For this review, take the finished solid that the model builds, in its own axes (mm). A direction names the side the tool comes from. Round coordinates to 2 decimals unless told otherwise and drop trailing zeros. Order: outer loops, then holes, each group sorted by start corner. A loop starts at its lowest first (then second) coordinate and runs counter-clockwise, first axis right, second up. Notation, with made-up numbers: (44, -32.75) -> (93, -32.75) arc R17 ccw to (93, -14.75) -> close; hole circle Ø7 at (60.25, 9). An arc over 180 degrees is marked (long way). Use a Markdown table: item, result. Add a question column.
1) Consider section D-D (x = 15.5). State the section outline as (y, z) points, plus the area to 3 significant figures.
2) Clearance check with flat-ended pins moving along their axes: P1, Ø10, axis at x = 23, y = -20, coming from the +Z side; P2, Ø5.5, axis at x = 19.5, z = 21, coming from the -Y side. State where each tip first meets the part, or that it passes through.
3) Consider section B-B (y = -3.5). State the section outline as (x, z) points.
4) Consider section C-C (x = 3). State the section outline as (y, z) points, plus the area to 3 significant figures.
5) Wall thickness on line 1 along X through (y, z) = (-9.5, 21); line 2 along Y through (x, z) = (29.5, 21); line 3 along Z through (x, y) = (30, -18.25): over which ranges is each line inside the solid? List them lowest first. Write a range as [from, to].
6) Draft analysis for pull direction X (two halves, no side actions). For faces 1 (the face through (19, -13, 0)), 2 (the face through (0, -10, 13)), 3 (the face through (12.7, -6, 25)), 4 (the face through (38.1, -10, 13)), state which applies: pulls with the +X half, pulls with the -X half, needs draft (parallel to the pull), parting line crosses it, or undercut.
7) Machinability: for faces 5 (the face through (19, -6, 19.05)), 6 (the face through (6, -6, 31.75)), 7 (the face through (19, -12.7, 18)), which of the approach directions +Z, -Z, +X, -X, +Y, -Y give a long, thin tool a straight path to every point of the face, cutting with its end or side? Answer none if there is none.
8) Consider section A-A (z = 30). State the section outline as (x, y) points.
```python
from build123d import *

# Parameters (mm, degrees)
F1_DEPTH = 38.1
F2_W     = 12.7
F2_H     = 12.7
F3_DEPTH = 228.6


with BuildPart() as f1:
    # F0 (on Right) → F1 (new body)
    with BuildSketch(Plane.YZ):
        Polygon((-25.4, 0), (0, 0), (0, 31.75), (-12.7, 31.75), (-12.7, 12.7), (-25.4, 12.7), align=None)
    extrude(amount=F1_DEPTH)

    # F2 (on Front) → F3 (cut)
    with BuildSketch(Plane.XZ):
        with Locations((19.05, 25.4)):
            Rectangle(F2_W, F2_H)
    extrude(amount=F3_DEPTH, mode=Mode.SUBTRACT)


solid = f1.part
```
Results list:
| question | item | result |
|---|---|---|
| 1 | outline | (-25.4, 0) -> (0, 0) -> (0, 19.05) -> (-12.7, 19.05) -> (-12.7, 12.7) -> (-25.4, 12.7) -> close |
| 1 | area | 403 mm2 |
| 2 | P1 | z = 12.7 |
| 2 | P2 | y = -12.7 |
| 3 | outline | (0, 0) -> (38.1, 0) -> (38.1, 31.75) -> (25.4, 31.75) -> (25.4, 19.05) -> (12.7, 19.05) -> (12.7, 31.75) -> (0, 31.75) -> close |
| 4 | outline | (-25.4, 0) -> (0, 0) -> (0, 31.75) -> (-12.7, 31.75) -> (-12.7, 12.7) -> (-25.4, 12.7) -> close |
| 4 | area | 565 mm2 |
| 5 | line 1 | [0, 12.7], [25.4, 38.1] |
| 5 | line 2 | [-12.7, 0] |
| 5 | line 3 | [0, 12.7] |
| 6 | face 1 | needs draft |
| 6 | face 2 | pulls with the -X half |
| 6 | face 3 | undercut |
| 6 | face 4 | pulls with the +X half |
| 7 | face 5 | +Z, +Y, -Y |
| 7 | face 6 | +Z, +X, -X, +Y, -Y |
| 7 | face 7 | +Z, +X, -X, -Y |
| 8 | outline | (0, -12.7) -> (12.7, -12.7) -> (12.7, 0) -> (0, 0) -> close; (25.4, -12.7) -> (38.1, -12.7) -> (38.1, 0) -> (25.4, 0) -> close |
